Check sheet for the drawn part. Datum: minimum x, y, z corner. Units: mm. A direction names the side the tool comes from. Give positions to 0.01 mm unless a question says otherwise; leave off trailing zeros. Order: outer loops, then holes, each group sorted by start corner. A loop starts at its lowest first (then second) coordinate and runs counter-clockwise, first axis right, second up. Notation, with made-up numbers: (28, 48) -> (36, 48) arc R13 cw to (36, 57) -> close; hole circle Ø6 at (2, 8.5). An arc over 180 degrees is marked (long way). Answer in a Markdown table with one row per item. Add a question column.
(1) Cross-section at A-A (z = 25). Record the cut outline in (x, y).
(2) Go/stop test with a flat-tipped pin: pin 1 (20 mm diameter, centred on x = 36.5, z = 29, fed in from +Y). Record where the tip stops, or that it passes through.
(3) Set-up check for the marked faces 5 and 6: record each of +Z, -Z, +X, -X, +Y, -Y from which the full face is reachable in a straight line by a thin tool's end or side.
(4) Cross-section at C-C (y = 11). Record the cut outline in (x, z).
(5) Cross-section at B-B (x = 41). Record the cut outline in (y, z), then the cut area to 3 significant figures.
(6) Thickness scan on L1, parallel to X at y = 3, z = 25; L2, parallel to Z at x = 78, y = 15.25; L3, parallel to X at y = 14.25, z = 36.5. Record the ranges inside material, lowest first. Write a range as [from, to].
(7) Cross-section at D-D (z = 13.5). Record the cut outline in (x, y), then the cut area to 4 significant figures.
(8) Release check for a two-part mould opening along Z. For the marked faces 1, 2, 3 and 4 record: released by +Z, released by -Z, zero draft, split by the parting line, or undercut.
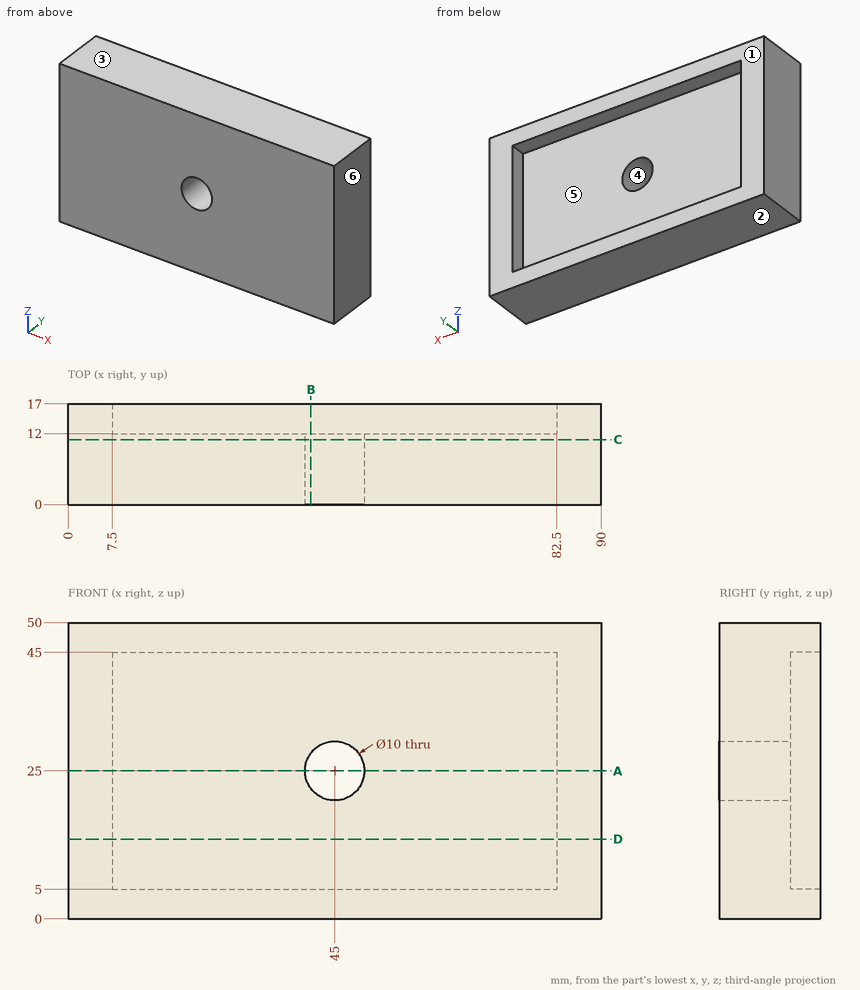
Answer below:
| question | item | result |
|---|---|---|
| 1 | outline | (0, 0) -> (40, 0) -> (40, 12) -> (7.5, 12) -> (7.5, 17) -> (0, 17) -> close; (50, 0) -> (90, 0) -> (90, 17) -> (82.5, 17) -> (82.5, 12) -> (50, 12) -> close |
| 2 | pin 1 | stops at y = 12 |
| 3 | face 5 | +Y |
| 3 | face 6 | +Z, -Z, +X, +Y, -Y |
| 4 | outline | (0, 0) -> (90, 0) -> (90, 50) -> (0, 50) -> close; hole circle Ø10 at (45, 25) |
| 5 | outline | (0, 0) -> (17, 0) -> (17, 5) -> (12, 5) -> (12, 22) -> (0, 22) -> close; (0, 28) -> (12, 28) -> (12, 45) -> (17, 45) -> (17, 50) -> (0, 50) -> close |
| 5 | area | 578 mm² |
| 6 | L1 | x = [0, 40], [50, 90] |
| 6 | L2 | z = [0, 5], [45, 50] |
| 6 | L3 | x = [0, 7.5], [82.5, 90] |
| 7 | outline | (0, 0) -> (90, 0) -> (90, 17) -> (82.5, 17) -> (82.5, 12) -> (7.5, 12) -> (7.5, 17) -> (0, 17) -> close |
| 7 | area | 1,155 mm² |
| 8 | face 1 | zero draft |
| 8 | face 2 | released by -Z |
| 8 | face 3 | released by +Z |
| 8 | face 4 | undercut |
